Here's the drawing with two shaded views (mm, measured from the low corner). I have some questions. A direction names the side the tool comes from. Coordinates: 2 decimals unless noted, no trailing zeros. Loops run counter-clockwise (first coordinate to the right, second up) from the corner with the lowest first, then second, coordinate; pieces in that order, holes last. Notation, with made-up numbers: (42.25, 68.25) -> (49.25, 68.25) arc R18 ccw to (49.25, 75.25) -> close; hole circle Ø8 at (51.25, 47). An arc over 180 degrees is marked (long way). Answer as a JSON object with one key per item and string values. Group by question number.
1) Which directions (+Z, -Z, +X, -X, +Y, -Y) give clear straight access to the entire face, cutting with the end or side of a thin tool? Please do the marked faces 4 and 5.
2) I need wall thicknesses on probe 1 along Z at (x, y) = (4.25, 1.85); probe 2 along Z at (x, y) = (4, 1.45) (1 decimal); probe 3 along X at (y, z) = (1.6, 4) (1 decimal). Which ranges of each line are inside material? Lowest first, please. Write a range as [from, to].
3) I want a section at C-C (z = 2.75). Write out the boundary of the cut face in (x, y) (1 decimal).
4) If we mould it in two halves opening along Z, with no side actions, what happens to the marked faces 1, 2 and 3? For each: +Z half, -Z half, draft (parallel to the pull), parting line (faces both ways), or undercut.
5) I'm going to push flat-ended pins straight in: pin 1 (1.6 mm diameter, centred on x = 1.44, z = 2.65, fed in from -Y); pin 2 (2 mm diameter, centred on x = 4.3, z = 4.3, fed in from -Y). Where does each tip first touch, or does it pass through?
6) I want a section at B-B (z = 7.75). Write out the boundary of the cut face in (x, y), then the cut area to 3 significant figures.
7) I want a section at D-D (y = 1.65). Write out the boundary of the cut face in (x, z).
8) I want a section at A-A (x = 4.3). Write out the boundary of the cut face in (y, z).
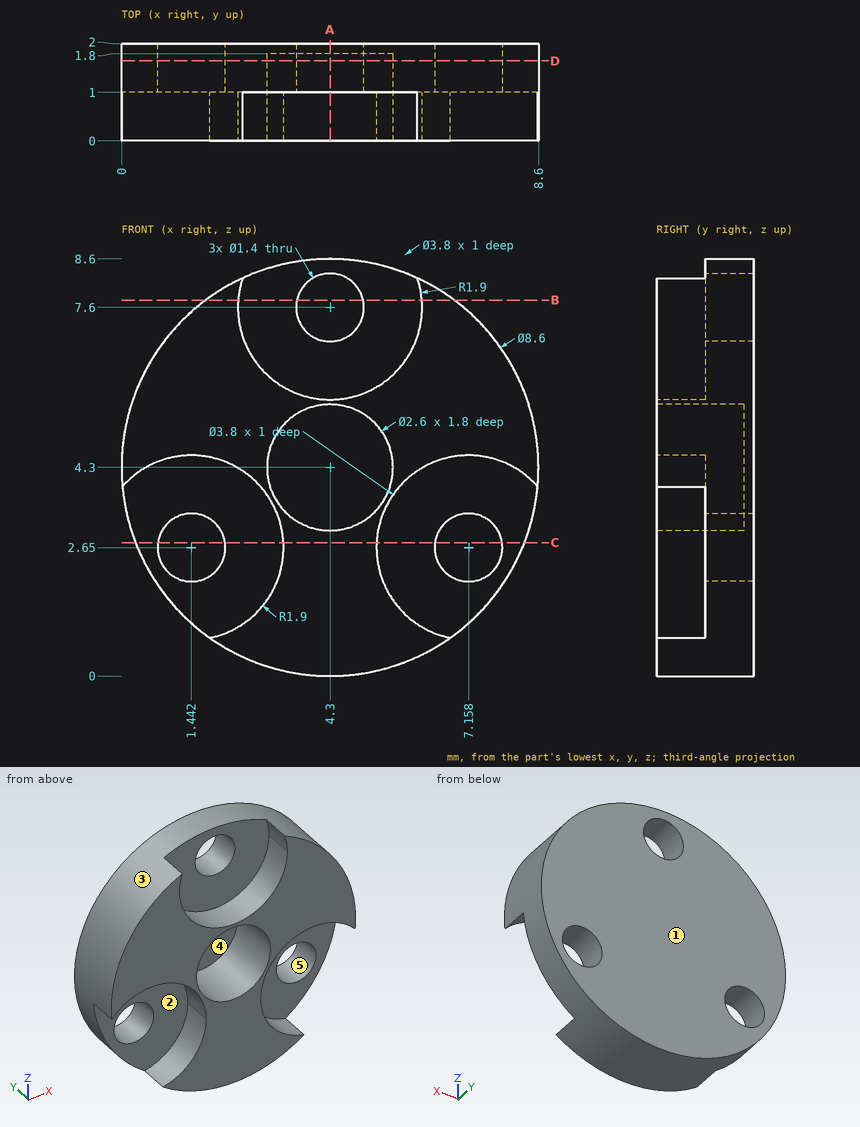
Determined:
{
 "1": {"face 4": "-Y", "face 5": "+Y, -Y"},
 "2": {"probe 1": "[0, 6.9], [8.3, 8.6]", "probe 2": "[0, 3], [5.6, 7], [8.2, 8.6]", "probe 3": "[0, 3], [5.6, 8.6]"},
 "3": {"outline": "(0.3, 1) -> (0.7, 1) -> (0.7, 2) -> (0.3, 2) -> close; (2.1, 1) -> (3.3, 1) -> (3.3, 0) -> (5.3, 0) -> (5.3, 1) -> (6.5, 1) -> (6.5, 2) -> (2.1, 2) -> close; (7.9, 1) -> (8.3, 1) -> (8.3, 2) -> (7.9, 2) -> close"},
 "4": {"face 1": "draft", "face 2": "undercut", "face 3": "parting line"},
 "5": {"pin 1": "y = 1", "pin 2": "y = 1.8"},
 "6": {"outline": "(1.73, 0) -> (2.41, 0) -> (2.41, 1) -> (3.62, 1) -> (3.62, 2) -> (1.73, 2) -> close; (4.98, 1) -> (6.19, 1) -> (6.19, 0) -> (6.87, 0) -> (6.87, 2) -> (4.98, 2) -> close", "area": "5.11 mm^2"},
 "7": {"outline": "circle Ø8.6 at (4.3, 4.3); hole circle Ø1.4 at (1.44, 2.65); hole circle Ø2.6 at (4.3, 4.3); hole circle Ø1.4 at (4.3, 7.6); hole circle Ø1.4 at (7.16, 2.65)"},
 "8": {"outline": "(0, 0) -> (2, 0) -> (2, 6.9) -> (1, 6.9) -> (1, 5.7) -> (0, 5.7) -> (0, 5.6) -> (1.8, 5.6) -> (1.8, 3) -> (0, 3) -> close; (1, 8.3) -> (2, 8.3) -> (2, 8.6) -> (1, 8.6) -> close"}
}
